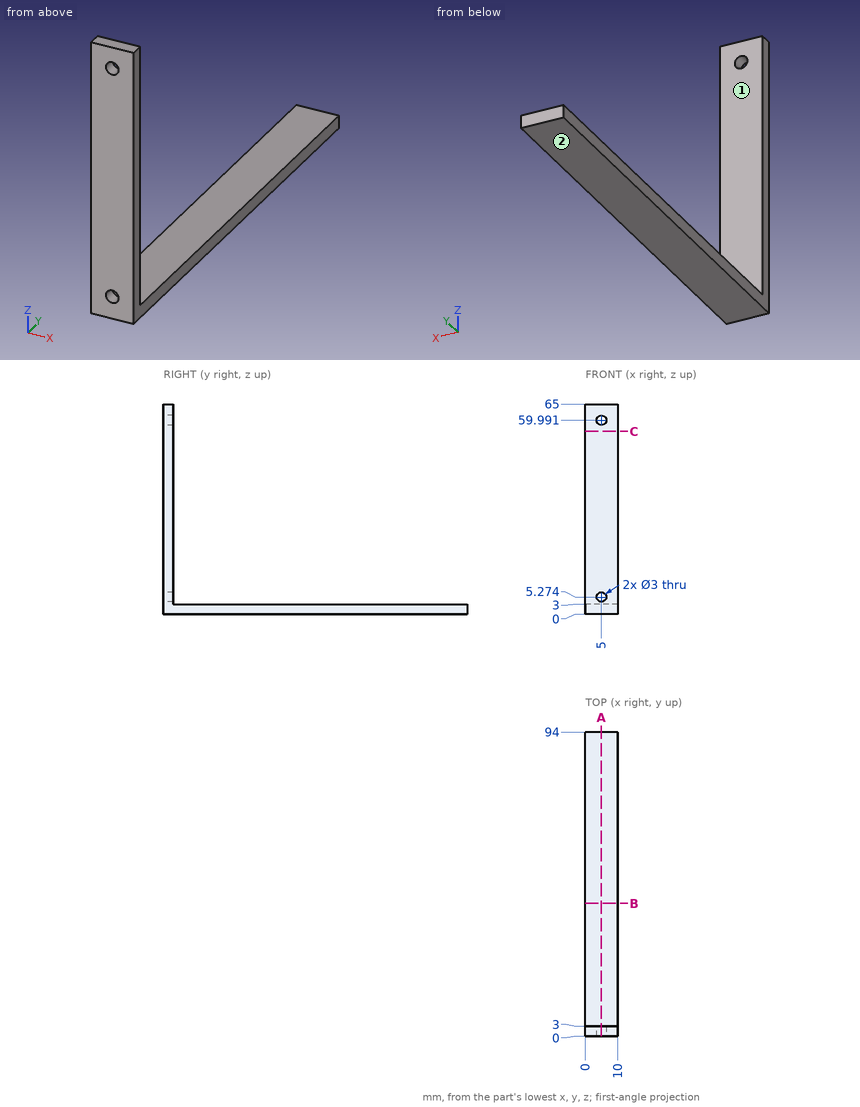
Source: three-view drawing plus pictorial views. Frame: mm from the lowest corner of the part. A direction names the side the tool comes from. Give positions to 0.01 mm unless a question says otherwise; leave off trailing zeros. Order: outer loops, then holes, each group sorted by start corner. A loop starts at its lowest first (then second) coordinate and runs counter-clockwise, first axis right, second up. Notation, with made-up numbers: (60.5, 19.25) -> (73.5, 19.25) arc R25 cw to (73.5, 35.25) -> close; hole circle Ø8 at (-35.5, 40). An arc over 180 degrees is marked (long way). Put each result on its own line as item: value.
Q1. Section B-B, the plane y = 41. Return loops of the section in (x, z).
Here are the results:
outline: (0, 0) -> (10, 0) -> (10, 3) -> (0, 3) -> close
Q2. Section A-A, the plane x = 5. Return loops of the section in (y, z).
Here are the results:
outline: (0, 0) -> (94, 0) -> (94, 3) -> (3, 3) -> (3, 3.77) -> (0, 3.77) -> close; (0, 6.77) -> (3, 6.77) -> (3, 58.49) -> (0, 58.49) -> close; (0, 61.49) -> (3, 61.49) -> (3, 65) -> (0, 65) -> close
Q3. Pin query (flat end, axial travel): pin 1 (6 mm diameter, centred on x = 2, z = 36, fed in from +Y). Return the tip coordinate at first contact, or that it passes through.
Here are the results:
pin 1: stops at y = 3
Q4. Material intervals for L1, parallel to Z at x = 5, y = 1.8; L2, parallel to Z at x = 1, y = 24.5, sorted ascending.
Here are the results:
L1: z = 0 to 3.77, 6.77 to 58.49, 61.49 to 65
L2: z = 0 to 3
Q5. Reachability of the marked faces 1 and 2 from +Z, -Z, +X, -X, +Y, -Y: full face, straight path, thin tool, end or side. Return the list, or none.
Here are the results:
face 1: +Z, +X, -X, +Y
face 2: -Z, +X, -X, +Y, -Y
